Autodesk Inventor part; units mm, degrees
ref_plane "Work Plane1" through (0, 0, 0) normal (0, 0, 1) x (1, 0, 0)
ref_plane "YZ Plane" through (0, 0, 0) normal (1, 0, 0) x (0, 1, 0)
ref_plane "XZ Plane" through (0, 0, 0) normal (0, 1, 0) x (-1, 0, 0)
sketch "Skizze" plane through (0, 0, 0) normal (1, 0, 0) x (0, 1, 0)
  circle A0 centre (0, 0) radius 12
  circle A1 centre (0, 0) radius 6.5
  dimension "d0" = 13
  dimension "d1" = 24
extrude "Körper" add sketch "Skizze" along normal blind 3
chamfer "Fase1" distance 0.5 angle 45 1 edges at (0, -12, 0) measured on face at (0, 9.9875, -1.4758)
chamfer "Fase2" distance 1.6 angle 45 1 edges at (0, -6.5, 0) measured on face at (0, 9.659, -1.4359)
ref_plane "Work Plane1" through (0, 0, 0) normal (0, 0, 1) x (1, 0, 0)
equation "\"d0\" = SD1"
equation "\"d1\" = SD2"
equation "\"d2\" = SD"
equation "\"d4\" = PHH"
equation "\"d5\" = FAWI"
equation "\"d10\" = PHH"
equation "\"d6\" = PHH1"
equation "\"d7\" = FAWI1"
equation "\"d11\" = PHH"
equation "\"SD1\" = 13"
equation "\"SD2\" = 24"
equation "\"SD\" = 3"
equation "\"FAWI\" = 45deg"
equation "\"FAWI1\" = 45deg"
equation "\"PHH\" = 0.5"
equation "\"PHH1\" = 1.6"
equation "\"NND\" = 12"
properties part number "DIN 6916 - 13" material "Stahl, weich"
The listing builds one solid part. Answer for the finished solid, in the listing's coordinates (mm). Give positions to 0.01 mm unless a question says otherwise; leave off trailing zeros. Order: outer loops, then holes, each group sorted by start corner. A loop starts at its lowest first (then second) coordinate and runs counter-clockwise, first axis right, second up.
Item 1: The part is cut by section C-C, the plane x = 2.1. Give the vertices of the cut face in (y, z).
From the geometry:
outline: circle Ø24 at (0, 0); hole circle Ø13 at (0, 0)
Item 2: For a pull along Z with two mould halves and no side action, classify faces 1 (the face through (2.29, -5.158, 3.955)), 2 (the face through (3, 5, -5)), 3 (the face through (1.73, -11.99, -0.53)) as pulls with the +Z half, pulls with the -Z half, needs draft (parallel to the pull), parting line crosses it, or undercut.
From the geometry:
face 1: undercut
face 2: needs draft
face 3: parting line crosses it
Item 3: Find the intervals of material crossed by probe 1 along Z at (x, y) = (2.35, 0); probe 2 along Y at (x, z) = (1.9, -2), in increasing order.
From the geometry:
probe 1: z = -12 to -6.5, 6.5 to 12
probe 2: y = -11.83 to -6.18, 6.18 to 11.83
Item 4: Given pin 1 Ø11.5 at (y, z) = (0, 0) entering from +X; pin 2 Ø1 at (x, z) = (1.5, -1) entering from +Y; pin 3 Ø1.5 at (x, y) = (2, -8.5) entering from -Z, each flat-ended and moving along its own axis, determine where each tip first touches the part or whether it passes through.
From the geometry:
pin 1: passes through
pin 2: stops at y = 11.99
pin 3: stops at z = -9.16
Item 5: The part is cut by section A-A, the plane z = 0. Give the vertices of the cut face in (x, y), and give its area (3 significant figures).
From the geometry:
outline: (0, -11.5) - (0.5, -12) - (3, -12) - (3, -6.5) - (1.6, -6.5) - (0, -8.1) - close; (0, 8.1) - (1.6, 6.5) - (3, 6.5) - (3, 12) - (0.5, 12) - (0, 11.5) - close
area: 30.2 mm2
